For this review, take the finished solid that the model builds, in its own axes (mm). A direction names the side the tool comes from. Round coordinates to 2 decimals unless told otherwise and drop trailing zeros. Order: outer loops, then holes, each group sorted by start corner. A loop starts at its lowest first (then second) coordinate and runs counter-clockwise, first axis right, second up. Notation, with made-up numbers: (34, 23.25) - (91, 23.25) arc R29 ccw to (91, 48.25) - close; hole circle Ø2 at (-22.5, 66.25). An arc over 180 degrees is marked (long way). Write each question's results on one line, items separated by ' | '. Start each with the question number.
(1) Take a section at B-B, the plane z = 0. Give the boundary of the cut face in (x, y) (3 decimals).
(2) For faces 4 (the flat face through (0, 39, -60.325)), 5 (the flat face through (288.925, -1, 0)), 6 (the cylindrical face through (-298.53, -1.57, -40.55)), 7 (the flat face through (-301.625, 26, -61)), list the 3-axis set-ups (+Z, -Z, +X, -X, +Y, -Y) from which the entire face can be reached by the end or side of a thin tool; tool diameter is ignored.
(3) For L1, parallel to Z at x = 218.5, y = 17 (3 decimals); L2, parallel to Y at x = 241, z = -33 (3 decimals), list the stretches that pass through material, from the lowest coordinate up. Write a range as from..to.
(4) Take a section at A-A, the plane x = -186.5. Give the boundary of the cut face in (y, z) (3 decimals), plus the area to 3 significant figures.
(5) Insertion check: pin 1 Ø5 at (x, z) = (-185.5, -22.5) entering from +Y; pin 2 Ø0.7 at (x, y) = (247, -2) entering from -Z; pin 3 Ø1 at (y, z) = (-2, 5.5) entering from -X (3 decimals). Each pin has a flat end and moves straight along its axis. Give the tip position at first contact, or say it passes through.
(6) Draft analysis for pull direction Z (two halves, no side actions). For faces 1 (the flat face through (-8, 38, 63.5)), 2 (the cylindrical face through (-298, 69.21, -61.89)), 3 (the cylindrical face through (-247.404, -1.565, -25.93)), state which applies: pulls with the +Z half, pulls with the -Z half, needs draft (parallel to the pull), parting line crosses it, or undercut.
```python
from build123d import *

# Parameters (mm, degrees)
SKETCH1_W                                 = 603.25
SKETCH1_H                                 = 127
BASE_FLANGE1_DEPTH                        = 3.175
EDGE_FLANGE1_STRIP_W                      = 19.05
EDGE_FLANGE1_STRIP_H                      = 3.175
EDGE_FLANGE1_STRIP_CUT_DEPTH              = 603.25
EDGE_FLANGE1_STRIP_2_W                    = 19.05
EDGE_FLANGE1_STRIP_2_H                    = 3.175
EDGE_FLANGE1_STRIP_CUT_2_DEPTH            = 603.25
EDGE_FLANGE1_DEPTH                        = 603.25
EDGE_FLANGE1_BEND_DEPTH                   = 603.25
F_1_4_CLEARANCE_HOLE1_D                   = 6.7564
HOLE_FOR_1_4_SELF_CLINCHING_NUTS_S_SS_C_D = 8.7376
CUT_EXTRUDE3_DEPTH                        = 336.319685151
FILLET1_R                                 = 6.35
HOLE_FOR_1_4_SELF_CLINCHING_NUTS_S_2_D    = 8.7376
CUT_EXTRUDE2_DEPTH                        = 318.515874603
FILLET3_R                                 = 12.7
FILLET4_R                                 = 12.7
F_1_4_START                               = -3.175
F_1_4_CLEARANCE_SLOT1_DEPTH               = 3.175
FILLET5_R                                 = 3.175


# Read off the part's stored shape, not the designer's step: 1/4 Clearance Slot1
# Sheet-metal steps are written as plain solids
with BuildPart() as part:
    # Sketch1 → Base-Flange1 (new body)
    with BuildSketch(Plane(origin=(0, 0, 0), x_dir=(1, 0, 0), z_dir=(0, 1, 0))):
        Rectangle(SKETCH1_W, SKETCH1_H)
    extrude(amount=-BASE_FLANGE1_DEPTH)

    # Edge-Flange1 strip (across the edge) → Edge-Flange1 strip cut (cut)
    with BuildSketch(Plane(origin=(301.625, 0, -63.5), x_dir=(0, 0, 1), z_dir=(-1, 0, 0))):
        with Locations((-3.175, -1.5875)):
            Rectangle(EDGE_FLANGE1_STRIP_W, EDGE_FLANGE1_STRIP_H)
    extrude(amount=EDGE_FLANGE1_STRIP_CUT_DEPTH, mode=Mode.SUBTRACT)

    # Edge-Flange1 strip 2 (across the edge) → Edge-Flange1 strip cut 2 (cut)
    with BuildSketch(Plane(origin=(-301.625, 0, 63.5), x_dir=(0, 0, -1), z_dir=(1, 0, 0))):
        with Locations((-3.175, -1.5875)):
            Rectangle(EDGE_FLANGE1_STRIP_2_W, EDGE_FLANGE1_STRIP_2_H)
    extrude(amount=EDGE_FLANGE1_STRIP_CUT_2_DEPTH, mode=Mode.SUBTRACT)

    # Edge-Flange1 section (across the edge) → Edge-Flange1 (add)
    with BuildSketch(Plane(origin=(301.625, 0, -63.5), x_dir=(0, 0, 1), z_dir=(-1, 0, 0))):
        with BuildLine():
            Line((0, 3.175), (0, 73.025))
            Line((0, 73.025), (3.175, 73.025))
            Line((3.175, 73.025), (3.175, 3.175))
            ThreePointArc((3.175, 3.175), (4.10493597, 0.92993597), (6.35, 0))
            Line((6.35, 0), (6.35, -3.175))
            ThreePointArc((6.35, -3.175), (1.859871939, -1.315128061), (0, 3.175))
        make_face()
    extrude(amount=EDGE_FLANGE1_DEPTH)

    # Edge-Flange1 section 2 (across the edge) → Edge-Flange1 bend (add)
    with BuildSketch(Plane(origin=(-301.625, 0, 63.5), x_dir=(0, 0, -1), z_dir=(1, 0, 0))):
        with BuildLine():
            Line((0, 3.175), (0, 73.025))
            Line((0, 73.025), (3.175, 73.025))
            Line((3.175, 73.025), (3.175, 3.175))
            ThreePointArc((3.175, 3.175), (4.10493597, 0.92993597), (6.35, 0))
            Line((6.35, 0), (6.35, -3.175))
            ThreePointArc((6.35, -3.175), (1.859871939, -1.315128061), (0, 3.175))
        make_face()
    extrude(amount=EDGE_FLANGE1_BEND_DEPTH)

    # 1/4 Clearance Hole1 (through all)
    with Locations(Plane.XY.offset(63.5)):
        with Locations((169.8625, 53.975), (185.7375, 53.975), (201.6125, 53.975), (217.4875, 53.975), (233.3625, 53.975), (249.2375, 53.975), (265.1125, 53.975), (280.9875, 53.975)):
            Hole(F_1_4_CLEARANCE_HOLE1_D / 2)

    # Hole for 1_4 Self-clinching Nuts _S_SS_C (through all)
    with Locations(Plane.XY.offset(63.5)):
        with Locations((-223.8375, 53.975)):
            Hole(HOLE_FOR_1_4_SELF_CLINCHING_NUTS_S_SS_C_D / 2)

    # Sketch33 → Cut-Extrude3 (cut, through all)
    with BuildSketch(Plane.XY.offset(63.5)):
        with BuildLine():
            Line((301.625, 73.025), (288.925, 73.025))
            Line((288.925, 73.025), (288.925, 64.147937825))
            ThreePointArc((288.925, 64.147937825), (293.8907, 53.975), (288.925, 43.802062175))
            Line((288.925, 43.802062175), (288.925, -3.175))
            Line((288.925, -3.175), (301.625, -3.175))
            Line((301.625, -3.175), (301.625, 73.025))
        make_face()
    extrude(amount=-CUT_EXTRUDE3_DEPTH, mode=Mode.SUBTRACT)

    # Fillet1
    fillet1_edges = [part.edges().sort_by_distance(p)[0] for p in [
        (288.925, 73.025, 61.9125),
        (288.925, 73.025, -61.9125),
    ]]
    fillet(fillet1_edges, radius=FILLET1_R)

    # Hole for 1_4 Self-clinching Nuts _S_ 2 (through all)
    with Locations(Plane.XY.offset(63.5)):
        with Locations((-273.05, 60.325), (-257.175, 17.4625), (-288.925, 17.4625)):
            Hole(HOLE_FOR_1_4_SELF_CLINCHING_NUTS_S_2_D / 2)

    # Sketch23 → Cut-Extrude2 (cut, through all)
    with BuildSketch(Plane.XZ.offset(3.175)):
        Polygon((-301.625, 38.1), (-244.475, 28.575), (-244.475, -28.575), (-301.625, -38.1), align=None)
    extrude(amount=-CUT_EXTRUDE2_DEPTH, mode=Mode.SUBTRACT)

    # Fillet3
    fillet3_edges = [part.edges().sort_by_distance(p)[0] for p in [
        (-301.625, -1.5875, -38.1),
        (-301.625, -1.5875, 38.1),
        (-244.475, -1.5875, 28.575),
        (-244.475, -1.5875, -28.575),
    ]]
    fillet(fillet3_edges, radius=FILLET3_R)

    # Fillet4
    fillet4_edges = [part.edges().sort_by_distance(p)[0] for p in [
        (-301.625, 73.025, -61.9125),
        (-301.625, 73.025, 61.9125),
    ]]
    fillet(fillet4_edges, radius=FILLET4_R)

    # 1/4 Clearance Slot1 outline → 1/4 Clearance Slot1 (cut)
    with BuildSketch(Plane(origin=(0, 0, 0), x_dir=(1, 0, 0), z_dir=(0, 1, 0)).offset(F_1_4_START)):
        with BuildLine():
            ThreePointArc((247.28805, -44.6532), (250.66625, -41.275), (247.28805, -37.8968))
            Line((247.28805, -37.8968), (246.42445, -37.8968))
            ThreePointArc((246.42445, -37.8968), (243.04625, -41.275), (246.42445, -44.6532))
            Line((246.42445, -44.6532), (247.28805, -44.6532))
        make_face()
        with BuildLine():
            ThreePointArc((-128.22555, -37.8968), (-131.60375, -41.275), (-128.22555, -44.6532))
            Line((-128.22555, -44.6532), (-127.36195, -44.6532))
            ThreePointArc((-127.36195, -44.6532), (-123.98375, -41.275), (-127.36195, -37.8968))
            Line((-127.36195, -37.8968), (-128.22555, -37.8968))
        make_face()
        with BuildLine():
            ThreePointArc((-127.36195, 37.8968), (-123.98375, 41.275), (-127.36195, 44.6532))
            Line((-127.36195, 44.6532), (-128.22555, 44.6532))
            ThreePointArc((-128.22555, 44.6532), (-131.60375, 41.275), (-128.22555, 37.8968))
            Line((-128.22555, 37.8968), (-127.36195, 37.8968))
        make_face()
        with BuildLine():
            ThreePointArc((246.42445, 44.6532), (243.04625, 41.275), (246.42445, 37.8968))
            Line((246.42445, 37.8968), (247.28805, 37.8968))
            ThreePointArc((247.28805, 37.8968), (250.66625, 41.275), (247.28805, 44.6532))
            Line((247.28805, 44.6532), (246.42445, 44.6532))
        make_face()
    extrude(amount=F_1_4_CLEARANCE_SLOT1_DEPTH, mode=Mode.SUBTRACT)

    # Fillet5
    fillet5_edges = [part.edges().sort_by_distance(p)[0] for p in [
        (288.925, 43.802062175, -61.9125),
        (288.925, 64.147937825, -61.9125),
        (288.925, 43.802062175, 61.9125),
        (288.925, 64.147937825, 61.9125),
    ]]
    fillet(fillet5_edges, radius=FILLET5_R)


solid = part.part
```
Results below:
1) outline: (-244.475, -3.175) - (288.925, -3.175) - (288.925, 0) - (-244.475, 0) - close
2) face 4: +X, -X, +Y | face 5: +Z, -Z, +X, -Y | face 6: -X, +Y, -Y | face 7: +Z, -Z, -X, +Y, -Y
3) L1: z = -63.5..-60.325, 60.325..63.5 | L2: y = -3.175..0
4) outline: (-3.175, -57.15) arc R6.35 ccw to (3.175, -63.5) - (73.025, -63.5) - (73.025, -60.325) - (3.175, -60.325) arc R3.175 cw to (0, -57.15) - (0, 57.15) arc R3.175 cw to (3.175, 60.325) - (73.025, 60.325) - (73.025, 63.5) - (3.175, 63.5) arc R6.35 ccw to (-3.175, 57.15) - close | area: 854 mm^2
5) pin 1: stops at y = 0 | pin 2: stops at z = -61.28 | pin 3: stops at x = -244.475
6) face 1: pulls with the +Z half | face 2: needs draft | face 3: undercut
